Autodesk Inventor part; units mm, degrees
ref_plane "YZ Plane" through (0, 0, 0) normal (1, 0, 0) x (0, 1, 0)
ref_plane "XZ Plane" through (0, 0, 0) normal (0, 1, 0) x (-1, 0, 0)
ref_plane "XY Plane" through (0, 0, 0) normal (0, 0, 1) x (1, 0, 0)
sketch "Skizze1" plane through (0, 0, 0) normal (0, 1, 0) x (-1, 0, 0)
  circle A0 centre (0, 0) radius 28
  circle A1 centre (0, 0) radius 30
  dimension "d0" = 56
  dimension "d1" = 60
extrude "Extrusion1" add sketch "Skizze1" along normal mid plane 10
sketch "Skizze2" plane through (0, 0, 0) normal (0, 1, 0) x (-1, 0, 0)
  circle A0 centre (0, 22.5) radius 3.25
  circle A1 centre (0, -22.5) radius 3.25
  line L0 (44.9262, 0) -> (-43.1306, 0) construction
  circle A2 centre (0, -22.5) radius 5
  circle A3 centre (0, 22.5) radius 5
  line L1 (0, 38.6377) -> (0, -60.2779) construction
  line L2 (3, 29.5) -> (-3, 29.5)
  line L3 (-3, 29.5) -> (-3, -29.5)
  line L4 (-3, -29.5) -> (3, -29.5)
  line L5 (3, -29.5) -> (3, 29.5)
  point P0 (0, 0)
  point P1 (-3, 26.5)
  point P2 (3, 26.5)
  point P3 (-3, -26.5)
  point P4 (3, -26.5)
  dimension "d4" = 45
  dimension "d5" = 6.5
  dimension "d6" = 6.5
  dimension "d7" = 10
  dimension "d8" = 10
  dimension "d9" = 6
  dimension "d21" = 59
extrude "Extrusion2" add sketch "Skizze2" along normal mid plane 5 contours A0 L5 A3 | A0 L3 A3 L5 | L5 A3 L3 A0 | A0 L3 A3 | A3 L3 L2 L5 | L5 A1 L3 A2 | A2 L5 A1 | L3 A1 A2 | L3 A1 L5 A2 | A2 L5 L4 L3
sketch "Skizze3" plane through (0, 0, 0) normal (0, 1, 0) x (-1, 0, 0)
  line L0 (-37.328, 53.3099) -> (47.5678, -67.9338) construction
  line L1 (48.5469, 69.3321) -> (-29.5635, -42.2211) construction
  line L2 (0, 56.0595) -> (0, -79.5026) construction
  circle A0 centre (0, 0) radius 30
  circle A1 centre (0, 0) radius 28
  line L3 (19.8236, 28.311) -> (13.732, 19.6114)
  line L4 (14.4871, -20.6897) -> (22.3283, -31.8882)
  point P0 (16.0601, -22.9363)
  point P1 (17.2073, -24.5746)
  point P2 (17.2073, 24.5746)
  point P3 (16.0601, 22.9363)
  dimension "d12" = 110
  dimension "d13" = 35
  dimension "d19" = 56
  dimension "d20" = 60
extrude "Extrusion3" cut sketch "Skizze3" along normal mid plane 10 contours A0 L4 A1 L3 picked at (29.0468, 2.3769)
sketch "Skizze4" plane through (0, 0, 0) normal (0, 1, 0) x (-1, 0, 0)
  line L0 (-8.0451, 13.9345) -> (38.1422, -66.0642) construction
  line L1 (17.2073, -24.5746) -> (16.0601, -22.9363) construction
  line L2 (0, 9.2259) -> (0, -51.7672) construction
  arc A0 (17.2073, 24.5746) -> (17.2073, -24.5746) centre (0, 0) ccw
  point P0 (16.6337, -23.7554)
  point P1 (15, -25.9808)
  point P2 (15, -25.9808)
  point P3 (19.2393, -22.9285)
  dimension "d16" = 30
ref_plane "Arbeitsebene3" through (-15.5, 0, -26.8468) normal (-0.4226, 0, -0.9063) x (0, -1, 0)
sketch "Skizze5" plane through (-15.5, 0, -26.8468) normal (-0.4226, 0, -0.9063) x (0, -1, 0)
  point P0 (0, -2.7018)
ref_plane "Arbeitsebene4" through (-15, 0, -25.9808) normal (-0.5, 0, -0.866) x (0, -1, 0)
sketch "Skizze6" plane through (-15, 0, -25.9808) normal (-0.5, 0, -0.866) x (0, -1, 0)
  circle A0 centre (0, 0) radius 2.5131
  point P0 (0, 0)
extrude "Extrusion5" cut sketch "Skizze6" against normal blind 1
mirror "Spiegeln2" about plane through (0, 0, 0) normal (0, 0, 1) of "Extrusion5"
fillet "Rundung1" radius 4 4 edges at (-16.6337, -5, -23.7554) (-16.6337, 5, -23.7554) (-16.6337, 5, 23.7554) (-16.6337, -5, 23.7554)
ref_plane "Arbeitsebene5" through (0, 0, 0) normal (0, 0, 1) x (1, 0, 0)
properties part number "_3D-Druck"
Could you check a few things on this model? Use its own coordinates, in mm. A direction names the side the tool comes from. Give positions to 0.01 mm unless a question says otherwise; leave off trailing zeros. Order: outer loops, then holes, each group sorted by start corner. A loop starts at its lowest first (then second) coordinate and runs counter-clockwise, first axis right, second up. Notation, with made-up numbers: (-25.75, 48) -> (16.25, 48) arc R17 cw to (16.25, 55) -> close; hole circle Ø8 at (16.5, 75.25). An arc over 180 degrees is marked (long way). Return JSON: item names as keys, results as strings.
1. For pin 1 Ø5 at (x, z) = (-2, 24.5) entering from +Y; pin 2 Ø1.1 at (y, z) = (-1, -27) entering from -X; pin 3 Ø1 at (x, y) = (23.5, -1.5) entering from +Z, each with a flat end and sliding along its axis, tell me the tip position at first contact or that it passes through.
Answer list:
{"pin 1": "stops at y = 2.5", "pin 2": "stops at x = -13.25", "pin 3": "stops at z = 19.26"}
2. Imagine slicing it at C-C on z = 0. List the corners of the cut face in (x, y) for me, then the cut area to 3 significant figures.
Answer list:
{"outline": "(28, -5) -> (30, -5) -> (30, 5) -> (28, 5) -> close", "area": "20.0 mm2"}
3. On a 3-axis mill with a long thin cutter (end or side, diameter ignored), from which of +Z, -Z, +X, -X, +Y, -Y can I reach the whole of each face in a straight line? I mean faces 1 (the flat face through (-2.2, -2.5, 25.2)), 2 (the flat face through (-16.498, -0.014, -23.562)), 3 (the flat face through (-3.3, 2.5, -23.8)), 4 (the flat face through (3, 0, 27)), 5 (the cylindrical face through (-15.626, 3.797, -24.305)). Say none if no direction works.
Answer list:
{"face 1": "-Y", "face 2": "-X, +Y, -Y", "face 3": "+Y", "face 4": "+Y, -Y", "face 5": "-X, +Y"}
4. Imagine slicing it at A-A on x = 0. List the corners of the cut face in (y, z) for me, then the cut area to 3 significant figures.
Answer list:
{"outline": "(-5, -30) -> (5, -30) -> (5, -28) -> (2.5, -28) -> (2.5, -25.75) -> (-2.5, -25.75) -> (-2.5, -28) -> (-5, -28) -> close; (-5, 28) -> (-2.5, 28) -> (-2.5, 25.75) -> (2.5, 25.75) -> (2.5, 28) -> (5, 28) -> (5, 30) -> (-5, 30) -> close; (-2.5, -19.25) -> (2.5, -19.25) -> (2.5, -17.5) -> (-2.5, -17.5) -> close; (-2.5, 17.5) -> (2.5, 17.5) -> (2.5, 19.25) -> (-2.5, 19.25) -> close", "area": "80.0 mm2"}
5. Imagine slicing it at D-D on x = 24. List the corners of the cut face in (y, z) for me, then the cut area to 3 significant figures.
Answer list:
{"outline": "(-5, -18) -> (5, -18) -> (5, -14.42) -> (-5, -14.42) -> close; (-5, 14.42) -> (5, 14.42) -> (5, 18) -> (-5, 18) -> close", "area": "71.6 mm2"}
6. Imagine slicing it at B-B on x = -10. List the corners of the cut face in (y, z) for me.
Answer list:
{"outline": "(-5, -28.28) -> (5, -28.28) -> (5, -26.15) -> (-5, -26.15) -> close; (-5, 26.15) -> (5, 26.15) -> (5, 28.28) -> (-5, 28.28) -> close"}
7. Thinking about a two-plate mould opening in X: for faces 6 (the cylindrical face through (-0.175, 0.035, -17.503)), 7 (the flat face through (28, -5, -4)), 8 (the cylindrical face through (-15.608, 3.797, 24.279)), which applies, pulls with the +X half, pulls with the -X half, needs draft (parallel to the pull), parting line crosses it, or undercut?
Answer list:
{"face 6": "undercut", "face 7": "needs draft", "face 8": "pulls with the -X half"}
8. I need wall thicknesses on line 1 (Z direction, x = 0, y = -0.1); line 2 (X direction, y = 1.3, z = -22.5); line 3 (Z direction, x = 0, y = 3). Which ranges of each line are inside material? Lowest first, please. Write a range as from..to.
Answer list:
{"line 1": "z = -30..-25.75, -19.25..-17.5, 17.5..19.25, 25.75..30", "line 2": "x = -5..-3.25, 3.25..5, 16.67..19.84", "line 3": "z = -30..-28, 28..30"}
